Can you work these out from the model? Positions are in its coordinate system, mm. Round coordinates to 2 decimals unless told otherwise and drop trailing zeros. Order: outer loops, then holes, each group sorted by start corner. A loop starts at its lowest first (then second) coordinate and runs counter-clockwise, first axis right, second up.
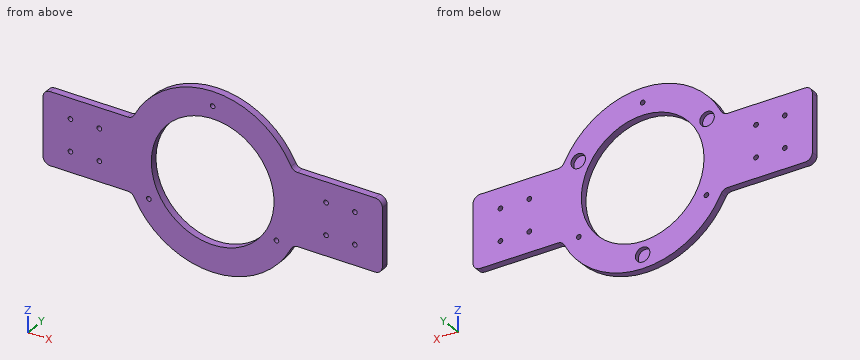
Autodesk Inventor part; units mm, degrees
ref_plane "YZ Plane" through (0, 0, 0) normal (1, 0, 0) x (0, 1, 0)
ref_plane "XZ Plane" through (0, 0, 0) normal (0, 1, 0) x (-1, 0, 0)
ref_plane "XY Plane" through (0, 0, 0) normal (0, 0, 1) x (1, 0, 0)
sketch "Sketch1" plane through (0, 0, 0) normal (0, 1, 0) x (-1, 0, 0)
  circle A0 centre (0, 0) radius 42.5
  arc A1 (55.6417, 25) -> (-55.6417, 25) centre (0, 0) ccw
  line L0 (0, 0) -> (0, -61)
  line L1 (0, 0) -> (0, 0)
  line L2 (0, 0) -> (0, -90.4875)
  line L3 (-117.5, 25) -> (-117.5, -25)
  line L4 (117.5, -25) -> (117.5, 25)
  line L5 (117.5, 25) -> (-117.5, -25) construction
  line L6 (-117.5, 25) -> (117.5, -25) construction
  line L7 (117.5, 25) -> (55.6417, 25)
  line L8 (-55.6417, 25) -> (-117.5, 25)
  line L9 (55.6417, -25) -> (117.5, -25)
  line L10 (-117.5, -25) -> (-55.6417, -25)
  arc A2 (-55.6417, -25) -> (55.6417, -25) centre (0, 0) ccw
  dimension "d0" = 85
  dimension "d29" = 61
  dimension "d46" = 235
  dimension "d47" = 50
extrude "Extrusion1" add sketch "Sketch1" along normal blind 5
sketch "Sketch2" plane through (0, 0, 0) normal (0, -1, 0) x (1, 0, 0)
  line L0 (-117.5, -25) -> (-117.5, 25)
  line L1 (-117.5, 0) -> (117.5, 0)
  line L2 (117.5, 25) -> (117.5, -25)
  arc A0 (55.6417, 25) -> (-55.6417, 25) centre (0, 0) ccw
  line L3 (0, 61) -> (0, -61)
  arc A1 (-55.6417, -25) -> (55.6417, -25) centre (0, 0) ccw
  circle A2 centre (-98.5, 11) radius 2
  line L4 (-117.5, 25) -> (-55.6417, 25)
  circle A3 centre (-78.5, 11) radius 2
  circle A4 centre (-98.5, -11) radius 2
  circle A5 centre (-78.5, -11) radius 2
  circle A6 centre (98.5, 11) radius 2
  circle A7 centre (78.5, 11) radius 2
  circle A8 centre (98.5, -11) radius 2
  circle A9 centre (78.5, -11) radius 2
  dimension "d51" = 4
  dimension "d52" = 19
  dimension "d53" = 14
  dimension "d54" = 4
  dimension "d55" = 20
hole "Hole1" at (-98.5, 0, 11) at (-78.5, 0, 11) at (-78.5, 0, -11) at (-98.5, 0, -11) at (78.5, 0, 11) at (98.5, 0, 11) at (98.5, 0, -11) at (78.5, 0, -11) direction (0, 1, 0) diameter 3.242 depth 11.8 tip angle 118
fillet "Fillet2" radius 5 8 edges at (-117.5, 2.5, -25) (-55.6417, 2.5, -25) (117.5, 2.5, -25) (55.6417, 2.5, -25) (117.5, 2.5, 25) (55.6417, 2.5, 25) (-55.6417, 2.5, 25) (-117.5, 2.5, 25)
sketch "Sketch4" plane through (0, 5, 0) normal (0, 1, 0) x (1, 0, 0)
  circle A0 centre (0, 0) radius 51.5
  point P0 (0, 51.5)
  point P1 (-44.6003, -25.75)
  point P2 (44.6003, -25.75)
  dimension "d57" = 103
  dimension "d60" = 360
hole "Pins" at (0, 5, -51.5) at (-44.6003, 5, 25.75) at (44.6003, 5, 25.75) direction (0, -1, 0) diameter 10 depth 3
sketch "Sketch5" plane through (0, 5, 0) normal (0, 1, 0) x (1, 0, 0)
  circle A0 centre (0, 0) radius 51
  point P0 (0, -51)
  point P1 (0, -51)
  dimension "d69" = 102
hole "Mounting Holes" at (0, 5, 51) direction (0, -1, 0) diameter 3.242 end through all
pattern_circular "Circular Pattern1" count 3 over 360 about axis through (0, -10, 0) along (0, 1, 0) of "Mounting Holes"
properties part number "Metal Head Thing"
(1) I'm going to push flat-ended pins straight in: pin 1 Ø3 at (x, y) = (-32.5, 1) entering from -Z; pin 2 Ø2 at (x, y) = (-55, 3) entering from +Z; pin 3 Ø3 at (x, z) = (43, 25) entering from +Y. Where does each tip first touch, or does it pass through?
(2) I want a section at C-C, the plane x = 19. List the corners of the cut face in (y, z) for me, plus the area to 3 significant figures.
(3) Please list where these lines run through material, in increasing order: probe 1 along Z at (x, y) = (0, 1.8); probe 2 along Z at (x, y) = (0, 2.45); probe 3 along Z at (x, y) = (78.5, 3.3).
(4) I want a section at B-B, the plane y = 1.2. Give the number of separate pieces and of enclosed holes in the cut face, plus the area to 3 significant figures.
(5) I want a section at A-A, the plane z = 0. List the corners of the cut face in (x, y) for me.
Ans:
1. pin 1: stops at z = -52.54
1. pin 2: stops at z = 28.37
1. pin 3: stops at y = 2
2. outline: (0, -57.97) - (5, -57.97) - (5, -38.02) - (0, -38.02) - close; (0, 38.02) - (5, 38.02) - (5, 57.97) - (0, 57.97) - close
2. area: 199 mm2
3. probe 1: z = -61 to -42.5, 42.5 to 49.38, 52.62 to 61
3. probe 2: z = -61 to -56.5, -46.5 to -42.5, 42.5 to 49.38, 52.62 to 61
3. probe 3: z = -25 to -12.62, -9.38 to 9.38, 12.62 to 25
4. separate pieces: 1
4. enclosed holes: 12
4. area: 11,700 mm2
5. outline: (-117.5, 0) - (-42.5, 0) - (-42.5, 5) - (-117.5, 5) - close; (42.5, 0) - (117.5, 0) - (117.5, 5) - (42.5, 5) - close
